Here's how the part is built. I have some questions about the finished solid (model axes, mm). A direction names the side the tool comes from. Round coordinates to 2 decimals unless told otherwise and drop trailing zeros. Write each loop counter-clockwise with the first axis right and the second up, starting at its lowest first coordinate (ties: lowest second). Pieces come first, ordered by that corner, then holes. Notation, with made-up numbers: (35.25, 79.25) - (63.25, 79.25) arc R20 cw to (63.25, 92.25) - close; hole circle Ø6 at (89.5, 69.5). An arc over 180 degrees is marked (long way). Return JSON: item names as keys, results as strings. Group by question number.
```python
from build123d import *

# Parameters (mm, degrees)
F1_DEPTH = 50.8
F2_W     = 25.4
F2_H     = 25.4
F3_DEPTH = 88.901


with BuildPart() as f1:
    # F0 (on Front) → F1 (new body)
    with BuildSketch(Plane.XZ):
        Polygon((-29.747168, 27.1924), (-42.447168, 27.1924), (-42.447168, -23.6076), (46.452832, -23.6076), (46.452832, 27.1924), (33.752832, 27.1924), (33.752832, -10.9076), (-29.747168, -10.9076), align=None)
    extrude(amount=F1_DEPTH)

    # F2 (on face) → F3 (cut, through all)
    with BuildSketch(Plane.YZ.offset(46.452832)):
        with Locations((-25.4, 8.1424)):
            Rectangle(F2_W, F2_H)
    extrude(amount=-F3_DEPTH, mode=Mode.SUBTRACT)


solid = f1.part
```
1) Imagine slicing it at C-C (z = 2). Please give me the cut outline in (x, y).
2) Imagine slicing it at B-B (y = -26). Please give me the cut outline in (x, z).
3) I need wall thicknesses on line 1 along X through (y, z) = (-11, 4.5); line 2 along Z through (x, y) = (38.5, -22); line 3 along Z through (x, y) = (17, -2). Which ranges of each line are inside material? Lowest first, please.
4) If we mould it in two halves opening along X, with no side actions, what happens to faces 4 (the flat face through (46.453, -25, -10)), 5 (the flat face through (-29.747, -25, -5)), 6 (the flat face through (1, -25, -23.608)), 7 (the flat face through (33.753, -25, 21))? For each: released by +X, released by -X, zero draft, split by the parting line, or undercut.
5) Imagine slicing it at A-A (x = -31.5). Please give me the cut outline in (y, z), plus the area to 3 significant figures.
6) Will this pin go through, and if not, where does the flat tip stop? pin 1 Ø6 at (x, y) = (-17, -34) entering from +Z.
7) For faces 1 (the flat face through (-36, -25, 27.192)), 2 (the flat face through (40, -38.1, 8)), 3 (the flat face through (2, -25, -10.908)), which set-ups out of +Z, -Z, +X, -X, +Y, -Y let a thin tool reach every point of the face, with its end or its side?
8) Imagine slicing it at D-D (y = -3.5). Please give me the cut outline in (x, z), plus the area to 3 significant figures.
Results found:
{
 "1": {"outline": "(-42.45, -50.8) - (-29.75, -50.8) - (-29.75, -38.1) - (-42.45, -38.1) - close; (-42.45, -12.7) - (-29.75, -12.7) - (-29.75, 0) - (-42.45, 0) - close; (33.75, -50.8) - (46.45, -50.8) - (46.45, -38.1) - (33.75, -38.1) - close; (33.75, -12.7) - (46.45, -12.7) - (46.45, 0) - (33.75, 0) - close"},
 "2": {"outline": "(-42.45, -23.61) - (46.45, -23.61) - (46.45, -4.56) - (33.75, -4.56) - (33.75, -10.91) - (-29.75, -10.91) - (-29.75, -4.56) - (-42.45, -4.56) - close; (-42.45, 20.84) - (-29.75, 20.84) - (-29.75, 27.19) - (-42.45, 27.19) - close; (33.75, 20.84) - (46.45, 20.84) - (46.45, 27.19) - (33.75, 27.19) - close"},
 "3": {"line 1": "x = -42.45 to -29.75, 33.75 to 46.45", "line 2": "z = -23.61 to -4.56, 20.84 to 27.19", "line 3": "z = -23.61 to -10.91"},
 "4": {"face 4": "released by +X", "face 5": "undercut", "face 6": "zero draft", "face 7": "undercut"},
 "5": {"outline": "(-50.8, -23.61) - (0, -23.61) - (0, 27.19) - (-50.8, 27.19) - close; hole (-38.1, -4.56) - (-12.7, -4.56) - (-12.7, 20.84) - (-38.1, 20.84) - close", "area": "1,940 mm²"},
 "6": {"pin 1": "stops at z = -10.91"},
 "7": {"face 1": "+Z, +X, -X, +Y, -Y", "face 2": "+X, -X", "face 3": "+Z, +Y, -Y"},
 "8": {"outline": "(-42.45, -23.61) - (46.45, -23.61) - (46.45, 27.19) - (33.75, 27.19) - (33.75, -10.91) - (-29.75, -10.91) - (-29.75, 27.19) - (-42.45, 27.19) - close", "area": "2,100 mm²"}
}
